Geometry: final body of the model. Coordinates: model frame, mm. Face numbers are marked on the shaded views. A direction names the side the tool comes from. Give positions to 0.01 mm unless a question says otherwise; leave off trailing zeros. Order: outer loops, then holes, each group sorted by start corner. A loop starts at its lowest first (then second) coordinate and runs counter-clockwise, first axis right, second up. Notation, with made-up numbers: (47, -35.75) - (87, -35.75) arc R23 ccw to (87, -0.75) - close; hole circle Ø3 at (5, -38.75). An arc over 180 degrees is marked (long way). Write item = value, one per line. Start each with the question number.
from build123d import *

# Parameters (mm, degrees)
BASPROSKE_W        = 5
BASPROSKE_H        = 10
TOOTHCUT_DEPTH     = 16
TEETHCUTS_COUNT    = 18
TEETHCUTS_ANGLE    = 340
BORSKE_R           = 2.5
BORE_DEPTH         = 50.0000508
SKETCH1_R          = 4.5
CUT_EXTRUDE1_DEPTH = 4


with BuildPart() as part:
    # BasProSke → Base-Revolve (revolve)
    with BuildSketch(Plane(origin=(0, 0, 0), x_dir=(1, 0, 0), z_dir=(0, 1, 0)), mode=Mode.PRIVATE) as base_revolve_sk:
        with Locations((2.5, 5)):
            Rectangle(BASPROSKE_W, BASPROSKE_H)
    revolve(base_revolve_sk.sketch.rotate(Axis((-10, 0, 0), (1, 0, 0)), 180), axis=Axis((-10, 0, 0), (1, 0, 0)))

    # TooCutSke → ToothCut (cut, through all)
    with BuildSketch(Plane(origin=(0, 0, 0), x_dir=(0, 0, -1), z_dir=(1, 0, 0))):
        with BuildLine():
            ThreePointArc((0.510641536, 7.732156635), (0, 7.749), (-0.510641536, 7.732156635))
            ThreePointArc((-0.510641536, 7.732156635), (-0.82619259, 8.907320741), (-1.515208602, 9.910236529))
            ThreePointArc((-1.515208602, 9.910236529), (0, 10.0254), (1.515208602, 9.910236529))
            ThreePointArc((1.515208602, 9.910236529), (0.82619259, 8.907320741), (0.510641536, 7.732156635))
        make_face()
    toothcut = extrude(amount=TOOTHCUT_DEPTH, mode=Mode.SUBTRACT)

    # TeethCuts: ToothCut ×18 about axis
    teethcuts_axis = Axis((-10, 0, 0), (1, 0, 0))
    for i in range(1, TEETHCUTS_COUNT):
        add(toothcut.rotate(teethcuts_axis, i * TEETHCUTS_ANGLE / (TEETHCUTS_COUNT - 1)), mode=Mode.SUBTRACT)

    # BorSke → Bore (cut, symmetric)
    with BuildSketch(Plane(origin=(0, 0, 0), x_dir=(0, 0, -1), z_dir=(1, 0, 0))):
        with Locations(Location((0, 0, 0), (0, 0, 180))):
            Circle(BORSKE_R)
    extrude(amount=BORE_DEPTH, both=True, mode=Mode.SUBTRACT)

    # Sketch1 → Cut-Extrude1 (cut)
    with BuildSketch(Plane(origin=(5, 0, 0), x_dir=(0, 0, -1), z_dir=(1, 0, 0))):
        Circle(SKETCH1_R)
    extrude(amount=-CUT_EXTRUDE1_DEPTH, mode=Mode.SUBTRACT)


solid = part.part
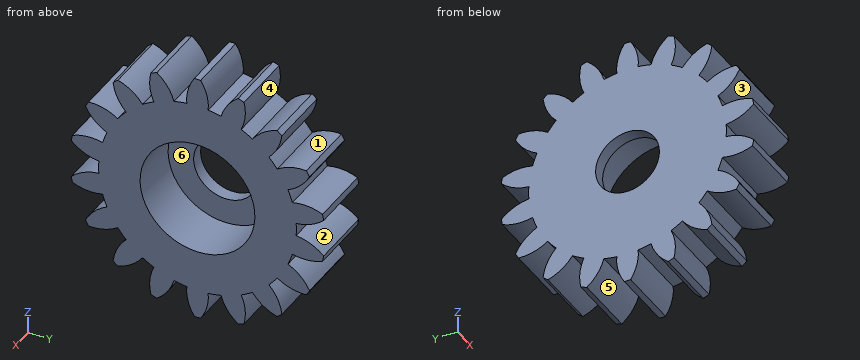
Q1. Section C-C, the plane y = -8. Return the cut outline in (x, z).
Q2. Material intervals for line 1 along Y through (x, z) = (0.75, 0); line 2 along Z through (x, y) = (1, -6); line 3 along X through (y, z) = (-3, 2.5), sorted ascending. Write a range as from..to.
Q3. Pull-direction query (Y, two-part tool) for the marked faces 1, 2 and 3; classes: +Y half, -Y half, draft (parallel to the pull), parting line (faces both ways), or undercut.
Q4. Contact query for flat-ended pins moving along their axis: pin 1 (3 mm diameter, centred on x = 2, y = 7.5, fed in from -Z); pin 2 (1.5 mm diameter, centred on x = 3, z = -5.5, fed in from +Y); pin 3 (1 mm diameter, centred on x = 4, y = -1, fed in from +Z). Output: stop coordinate, or through.
Q5. Set-up query: the marked faces 4, 5 and 6. Return all of +Z, -Z, +X, -X, +Y, -Y with unobstructed straight access to the full face (end or side cutting, diameter ignored); none if empty.
Q6. Section D-D, the plane y = 8.25. Return the cut outline in (x, z), then the cut area to 3 significant figures.
Q7. Section A-A, the plane z = 0. Return the cut outline in (x, y), then the cut area to 3 significant figures.
Q8. Section B-B, the plane y = 0. Return the cut outline in (x, z).
The answers:
q1.outline = (0, -5.21) - (5, -5.21) - (5, -3.74) - (0, -3.74) - close; (0, -2.27) - (5, -2.27) - (5, -0.55) - (0, -0.55) - close; (0, 0.55) - (5, 0.55) - (5, 2.27) - (0, 2.27) - close; (0, 3.74) - (5, 3.74) - (5, 5.21) - (0, 5.21) - close
q2.line_1 = -7.75..-2.5, 2.5..7.75
q2.line_2 = -7.74..-5.85, -4.9..4.9, 5.85..7.74
q2.line_3 = 0..1
q3.face_1 = undercut
q3.face_2 = +Y half
q3.face_3 = -Y half
q4.pin_1 = -7.82
q4.pin_2 = 8.78
q4.pin_3 = 9.55
q5.face_4 = +X, -X
q5.face_5 = -Z, +X, -X
q5.face_6 = +X
q6.outline = (0, -5.22) - (5, -5.22) - (5, -3.99) - (0, -3.99) - close; (0, -2.28) - (5, -2.28) - (5, -0.6) - (0, -0.6) - close; (0, 0.6) - (5, 0.6) - (5, 2.28) - (0, 2.28) - close; (0, 3.99) - (5, 3.99) - (5, 5.22) - (0, 5.22) - close
q6.area = 29.1 mm²
q7.outline = (0, -7.75) - (5, -7.75) - (5, -4.5) - (1, -4.5) - (1, -2.5) - (0, -2.5) - close; (0, 2.5) - (1, 2.5) - (1, 4.5) - (5, 4.5) - (5, 7.75) - (0, 7.75) - close
q7.area = 36.5 mm²
q8.outline = (0, -10) - (5, -10) - (5, -4.5) - (1, -4.5) - (1, -2.5) - (0, -2.5) - close; (0, 2.5) - (1, 2.5) - (1, 4.5) - (5, 4.5) - (5, 10) - (0, 10) - close
